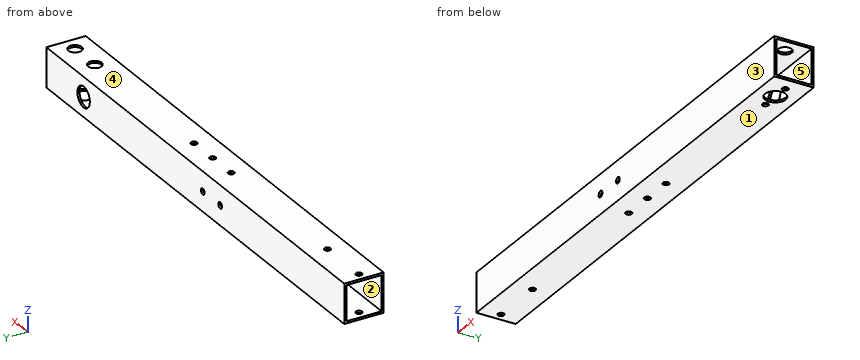
```python
from build123d import *

# Parameters (mm, degrees)
SKETCH1_W           = 19
SKETCH1_H           = 19
SKETCH1_W_2         = 17
SKETCH1_H_2         = 17
BOSS_EXTRUDE1_DEPTH = 240
SKETCH3_R           = 1.5
CUT_EXTRUDE1_DEPTH  = 241.938270103
SKETCH7_R           = 1.5
CUT_EXTRUDE5_DEPTH  = 241.938270103
SKETCH9_R           = 5
CUT_EXTRUDE6_DEPTH  = 10
SKETCH10_R          = 3.25
CUT_EXTRUDE7_DEPTH  = 10
SKETCH11_R          = 5
SKETCH11_R_2        = 1.5
CUT_EXTRUDE8_DEPTH  = 10


with BuildPart() as part:
    # Sketch1 → Boss-Extrude1 (new body)
    with BuildSketch(Plane(origin=(0, 0, 0), x_dir=(0, 0, -1), z_dir=(1, 0, 0))):
        Rectangle(SKETCH1_W, SKETCH1_H)
        Rectangle(SKETCH1_W_2, SKETCH1_H_2, mode=Mode.SUBTRACT)
    extrude(amount=BOSS_EXTRUDE1_DEPTH)

    # Sketch3 → Cut-Extrude1 (cut, through all)
    with BuildSketch(Plane.XY.offset(9.5)):
        with Locations((4, 0)):
            Circle(SKETCH3_R)
        with Locations((29.4, 0)):
            Circle(SKETCH3_R)
        with Locations((106.9, 0)):
            Circle(SKETCH3_R)
        with Locations((121.9, 0)):
            Circle(SKETCH3_R)
        with Locations((136.9, 0)):
            Circle(SKETCH3_R)
    extrude(amount=-CUT_EXTRUDE1_DEPTH, mode=Mode.SUBTRACT)

    # Sketch7 → Cut-Extrude5 (cut, through all)
    with BuildSketch(Plane(origin=(0, 9.5, 0), x_dir=(1, 0, 0), z_dir=(0, 1, 0))):
        with Locations(Location((100, 0, 0), (0, 0, 270))):
            Circle(SKETCH7_R)
        with Locations(Location((114, 0, 0), (0, 0, 270))):
            Circle(SKETCH7_R)
    extrude(amount=-CUT_EXTRUDE5_DEPTH, mode=Mode.SUBTRACT)

    # Sketch9 → Cut-Extrude6 (cut)
    with BuildSketch(Plane(origin=(0, 9.5, 0), x_dir=(1, 0, 0), z_dir=(0, 1, 0))):
        with Locations(Location((210, 0, 0), (0, 0, 270))):
            Circle(SKETCH9_R)
    extrude(amount=-CUT_EXTRUDE6_DEPTH, mode=Mode.SUBTRACT)

    # Sketch10 → Cut-Extrude7 (cut)
    with BuildSketch(Plane.XY.offset(9.5)):
        with Locations((232.75, 0)):
            Circle(SKETCH10_R)
        with Locations((216.75, 0)):
            Circle(SKETCH10_R)
    extrude(amount=-CUT_EXTRUDE7_DEPTH, mode=Mode.SUBTRACT)

    # Sketch11 → Cut-Extrude8 (cut)
    with BuildSketch(Plane(origin=(0, 0, -9.5), x_dir=(-1, 0, 0), z_dir=(0, 0, -1))):
        with Locations((-225, 0)):
            Circle(SKETCH11_R)
        with Locations((-217, 0)):
            Circle(SKETCH11_R_2)
        with Locations((-233, 0)):
            Circle(SKETCH11_R_2)
    extrude(amount=-CUT_EXTRUDE8_DEPTH, mode=Mode.SUBTRACT)


solid = part.part
```
Source: CAD feature listing. Evaluate the final solid. Frame: model axes, mm. Face numbers are marked on the shaded views. A direction names the side the tool comes from. Coordinates: 2 decimals unless noted, no trailing zeros. Write each loop counter-clockwise with the first axis right and the second up, starting at its lowest first coordinate (ties: lowest second). Pieces come first, ordered by that corner, then holes. Notation, with made-up numbers: M -30.75,13 L -4.75,13 A24 ccw -4.75,26 Z; hole C 83.5,67 d2. An arc over 180 degrees is marked long. Answer as a JSON object with one key per item and string values.
1. Cut plane A-A on x = 78. Output: boundary loops of the cut face in (y, z), plus the area to 3 significant figures.
Evaluation:
{"outline": "M -9.5,-9.5 L 9.5,-9.5 L 9.5,9.5 L -9.5,9.5 Z; hole M -8.5,-8.5 L 8.5,-8.5 L 8.5,8.5 L -8.5,8.5 Z", "area": "72.0 mm^2"}
2. Ray query, L1, parallel to X at y = 9.15, z = 0; L2, parallel to Y at x = 209, z = -7.5. Return the intervals inside material, ascending.
Evaluation:
{"L1": "0 to 98.5, 101.5 to 112.5, 115.5 to 205, 215 to 240", "L2": "-9.5 to -8.5, 8.5 to 9.5"}
3. Cut plane B-B on x = 225. Output: boundary loops of the cut face in (y, z).
Evaluation:
{"outline": "M -9.5,-9.5 L -5,-9.5 L -5,-8.5 L -8.5,-8.5 L -8.5,8.5 L 8.5,8.5 L 8.5,-8.5 L 5,-8.5 L 5,-9.5 L 9.5,-9.5 L 9.5,9.5 L -9.5,9.5 Z"}
4. Draft query along Z for the marked faces 3, 4 and 5. Return one class per face: released by +Z, released by -Z, zero draft, split by the parting line, or undercut.
Evaluation:
{"face 3": "zero draft", "face 4": "released by +Z", "face 5": "undercut"}
5. Contact query for a flat-ended pin moving along its axis: P1, Ø1.8, axis at x = 114, z = 0, coming from the +Y side. Output: stop coordinate, or through.
Evaluation:
{"P1": "through"}
6. Access query for the marked faces 1 and 2. Directions: +Z, -Z, +X, -X, +Y, -Y. A direction counts if a zero-diameter tool reaches every point of the face in a straight line with its end or side. Return the directions, or none.
Evaluation:
{"face 1": "-Z, +X, -X, +Y, -Y", "face 2": "+X, -X"}
